```python
from build123d import *
from OCP.BRepFilletAPI import BRepFilletAPI_MakeChamfer

# Parameters (mm, degrees)
BOSS_EXTRUDE1_DEPTH = 9.8
CUT_EXTRUDE1_START  = -4.1
CUT_EXTRUDE1_DEPTH  = 4.1
SKETCH3_W           = 60.6
SKETCH3_H           = 100.9
CUT_EXTRUDE2_DEPTH  = 6.3
SKETCH4_W           = 1.6
SKETCH4_H           = 58.7
SKETCH4_W_2         = 45.4
SKETCH4_H_2         = 71.1
CUT_EXTRUDE3_DEPTH  = 71.319005255
BOSS_EXTRUDE3_START = -4.5
BOSS_EXTRUDE3_DEPTH = 4.5
CUT_EXTRUDE4_START  = -2.5
CUT_EXTRUDE4_DEPTH  = 4
CUT_EXTRUDE5_START  = -1.7
CUT_EXTRUDE5_DEPTH  = 3.1
FILLET1_R           = 6
FILLET2_R           = 4
FILLET3_R           = 2.5
CUT_EXTRUDE6_DEPTH  = 1.5
CHAMFER1_SIZE       = 1
CHAMFER2_SIZE       = 0.6
CHAMFER2_SIZE2      = 0.651920241
CHAMFER2_SIZE2_2    = 0.691050664
FILLET4_R           = 2


# Read off the part's stored shape, not the designer's step: Boss-Extrude3
with BuildPart() as part:
    # Sketch1 → Boss-Extrude1 (new body)
    with BuildSketch(Plane.XY):
        with BuildLine():
            ThreePointArc((-38, 0), (-37.524874157, -29.190462912), (-36.1, -58.35))
            Line((-36.1, -58.35), (36.1, -58.35))
            ThreePointArc((36.1, -58.35), (37.524874157, -29.190462912), (38, 0))
            ThreePointArc((38, 0), (37.524874157, 29.190462912), (36.1, 58.35))
            Line((36.1, 58.35), (-36.1, 58.35))
            ThreePointArc((-36.1, 58.35), (-37.524874157, 29.190462912), (-38, 0))
        make_face()
    extrude(amount=BOSS_EXTRUDE1_DEPTH)

    # Sketch2 → Cut-Extrude1 (cut)
    with BuildSketch(Plane.XY.offset(9.8).offset(CUT_EXTRUDE1_START)):
        with BuildLine():
            ThreePointArc((36.1, -58.35), (38, 0), (36.1, 58.35))
            Line((36.1, 58.35), (-36.1, 58.35))
            ThreePointArc((-36.1, 58.35), (-38, 0), (-36.1, -58.35))
            Line((-36.1, -58.35), (36.1, -58.35))
        make_face()
        with BuildLine():
            Line((-32, 54.5), (32, 54.5))
            ThreePointArc((32, 54.5), (33.8, 0), (32, -54.5))
            Line((32, -54.5), (-32, -54.5))
            ThreePointArc((-32, -54.5), (-33.8, 0), (-32, 54.5))
        make_face(mode=Mode.SUBTRACT)
    extrude(amount=CUT_EXTRUDE1_DEPTH, mode=Mode.SUBTRACT)

    # Sketch3 → Cut-Extrude2 (cut)
    with BuildSketch(Plane.XY.offset(9.8)):
        with Locations((0, 0.65)):
            Rectangle(SKETCH3_W, SKETCH3_H)
    extrude(amount=-CUT_EXTRUDE2_DEPTH, mode=Mode.SUBTRACT)

    # Sketch4 → Cut-Extrude3 (cut, through all)
    with BuildSketch(Plane(origin=(0, 0, 0), x_dir=(-1, 0, 0), z_dir=(0, 0, -1))):
        with Locations((23.5, -3)):
            Rectangle(SKETCH4_W, SKETCH4_H)
        with Locations((0, 0.1)):
            Rectangle(SKETCH4_W_2, SKETCH4_H_2)
        with BuildLine():
            Line((-2.1, -43.35), (2.1, -43.35))
            ThreePointArc((2.1, -43.35), (3.8, -41.65), (2.1, -39.95))
            Line((2.1, -39.95), (-2.1, -39.95))
            ThreePointArc((-2.1, -39.95), (-3.8, -41.65), (-2.1, -43.35))
        make_face()
        with BuildLine():
            Line((1.7, 39.85), (1.7, 44.05))
            ThreePointArc((1.7, 44.05), (0, 45.75), (-1.7, 44.05))
            Line((-1.7, 44.05), (-1.7, 39.85))
            ThreePointArc((-1.7, 39.85), (0, 38.15), (1.7, 39.85))
        make_face()
    extrude(amount=-CUT_EXTRUDE3_DEPTH, mode=Mode.SUBTRACT)

    # Boss-Extrude3 outline → Boss-Extrude3 (add)
    with BuildSketch(Plane(origin=(0, 54.5, 0), x_dir=(1, 0, 0), z_dir=(0, 1, 0)).offset(BOSS_EXTRUDE3_START)):
        Polygon((0, -3.5), (0, -9.8), (5.5, -9.8), (6, -15), (22, -15), (22.5, -9.8), (26, -9.8), (26, -3.5), align=None)
    boss_extrude3 = extrude(amount=BOSS_EXTRUDE3_DEPTH)

    # Sketch7 → Cut-Extrude4 (cut)
    with BuildSketch(Plane(origin=(0, 54.5, 0), x_dir=(1, 0, 0), z_dir=(0, 1, 0)).offset(CUT_EXTRUDE4_START)):
        Polygon((19.5, -14), (8.5, -14), (7.346153846, 1), (20.653846154, 1), align=None)
    cut_extrude4 = extrude(amount=CUT_EXTRUDE4_DEPTH, mode=Mode.SUBTRACT)

    # Mirror3: Boss-Extrude3, Cut-Extrude4 across plane
    add(boss_extrude3.mirror(Plane(origin=(0, 0, 0), x_dir=(0, 0, 1), z_dir=(1, 0, 0))))
    add(cut_extrude4.mirror(Plane(origin=(0, 0, 0), x_dir=(0, 0, 1), z_dir=(1, 0, 0))), mode=Mode.SUBTRACT)

    # Sketch8 → Cut-Extrude5 (cut)
    with BuildSketch(Plane.XZ.offset(54.5).offset(CUT_EXTRUDE5_START)):
        Polygon((-20.75, -1), (-19.6, 8.2), (-8.4, 8.2), (-7.25, -1), align=None)
    cut_extrude5 = extrude(amount=CUT_EXTRUDE5_DEPTH, mode=Mode.SUBTRACT)

    # Mirror4: Cut-Extrude5 across plane
    add(cut_extrude5.mirror(Plane(origin=(0, 0, 0), x_dir=(0, 0, 1), z_dir=(1, 0, 0))), mode=Mode.SUBTRACT)

    # Fillet1
    fillet1_edges = [part.edges().sort_by_distance(p)[0] for p in [
        (36.1, 58.35, 2.85),
        (36.1, -58.35, 2.85),
        (-36.1, -58.35, 2.85),
        (-36.1, 58.35, 2.85),
    ]]
    fillet(fillet1_edges, radius=FILLET1_R)

    # Fillet2
    fillet2_edges = [part.edges().sort_by_distance(p)[0] for p in [
        (-30.3, -49.8, 6.65),
        (-30.3, 51.1, 6.65),
        (30.3, 51.1, 6.65),
        (30.3, -49.8, 6.65),
    ]]
    fillet(fillet2_edges, radius=FILLET2_R)

    # Fillet3
    fillet3_edges = [part.edges().sort_by_distance(p)[0] for p in [
        (32, 54.5, 7.75),
        (-32, 54.5, 7.75),
        (-32, -54.5, 7.75),
        (32, -54.5, 7.75),
    ]]
    fillet(fillet3_edges, radius=FILLET3_R)

    # Sketch10 → Cut-Extrude6 (cut)
    with BuildSketch(Plane.XY.offset(5.7)):
        with BuildLine():
            Line((30.460657239, 55.35), (-30.460657239, 55.35))
            ThreePointArc((-30.460657239, 55.35), (-32.518710973, 54.532753955), (-33.455473858, 52.526276553))
            ThreePointArc((-33.455473858, 52.526276553), (-35, 0), (-33.455473858, -52.526276553))
            ThreePointArc((-33.455473858, -52.526276553), (-33.188926222, -53.597617073), (-32.552904835, -54.5))
            Line((-32.552904835, -54.5), (-34.974801677, -54.5))
            ThreePointArc((-34.974801677, -54.5), (-35.303180702, -53.59497651), (-35.45201827, -52.643794255))
            ThreePointArc((-35.45201827, -52.643794255), (-37, 0), (-35.45201827, 52.643794255))
            ThreePointArc((-35.45201827, 52.643794255), (-33.890746795, 55.987923259), (-30.460657239, 57.35))
            Line((-30.460657239, 57.35), (30.460657239, 57.35))
            ThreePointArc((30.460657239, 57.35), (33.890746795, 55.987923259), (35.45201827, 52.643794255))
            ThreePointArc((35.45201827, 52.643794255), (37, 0), (35.45201827, -52.643794255))
            ThreePointArc((35.45201827, -52.643794255), (35.303180702, -53.59497651), (34.974801677, -54.5))
            Line((34.974801677, -54.5), (32.552904835, -54.5))
            ThreePointArc((32.552904835, -54.5), (33.188926222, -53.597617073), (33.455473858, -52.526276553))
            ThreePointArc((33.455473858, -52.526276553), (35, 0), (33.455473858, 52.526276553))
            ThreePointArc((33.455473858, 52.526276553), (32.518710973, 54.532753955), (30.460657239, 55.35))
        make_face()
    extrude(amount=-CUT_EXTRUDE6_DEPTH, mode=Mode.SUBTRACT)

    # Chamfer1
    # the kernel refuses this chamfer: 1 mm, written as the material it takes off along each edge
    with BuildSketch(Plane(origin=(32.228209132, -54.5, 9.8), x_dir=(0, 0.9996219169112968, 0.02749587661058555), z_dir=(-1, 0, 0))) as chamfer1_piece_1:
        Polygon((CHAMFER1_SIZE * 0.999621916911, CHAMFER1_SIZE * 0.0274958766106), (-CHAMFER1_SIZE * 0.0274958766106, CHAMFER1_SIZE * 0.999621916911), (0, 0), align=None)
    extrude(amount=64.456418264, mode=Mode.SUBTRACT)

    # Chamfer2: one chamfer whose edges measure the first distance from different faces: ONE call of the kernel's chamfer builder (chamfer() names one face for all edges)
    chamfer2_edges_1 = [part.edges().sort_by_distance(p)[0] for p in [
        (14, 52, 0),
        (14, 56, 0),
        (-14, 52, 0),
        (-14, 56, 0),
        (-14, -52.8, 0),
        (-14, -55.9, 0),
        (14, -52.8, 0),
        (14, -55.9, 0),
        (0, -58.35, 0),
        (0, 58.35, 0),
        (38, 0, 0),
        (-38, 0, 0),
        (34.576764706, 56.715507911, 0),
        (-34.576764706, 56.715507911, 0),
        (34.576764706, -56.715507911, 0),
        (-34.576764706, -56.715507911, 0),
        (1.7, 41.95, 0),
        (-1.7, 41.95, 0),
        (0, 45.75, 0),
        (0, 38.15, 0),
        (0, -39.95, 0),
        (0, -43.35, 0),
        (-3.8, -41.65, 0),
        (3.8, -41.65, 0),
        (-23.5, -32.35, 0),
        (-22.7, -33.9, 0),
        (0, 35.65, 0),
        (-22.7, 31, 0),
        (-23.5, 26.35, 0),
        (-24.3, -3, 0),
        (22.7, 0.1, 0),
        (0, -35.45, 0),
    ]]
    chamfer2_edges_2 = [part.edges().sort_by_distance(p)[0] for p in [
        (20.576923077, 54, 0),
        (7.423076923, 54, 0),
    ]]
    chamfer2_side_2 = [part.faces().sort_by_distance(p)[0] for p in [
        (0, -56.957344623, 0),
    ]]
    chamfer2_edges_3 = [part.edges().sort_by_distance(p)[0] for p in [
        (-20.576923077, 54, 0),
    ]]
    chamfer2_side_3 = [part.faces().sort_by_distance(p)[0] for p in [
        (-20.098958851, 53.596109806, 6.213534938),
    ]]
    chamfer2_edges_4 = [part.edges().sort_by_distance(p)[0] for p in [
        (-7.423076923, 54, 0),
    ]]
    chamfer2_side_4 = [part.faces().sort_by_distance(p)[0] for p in [
        (-7.901041149, 53.596109806, 6.213534938),
    ]]
    chamfer2_edges_5 = [part.edges().sort_by_distance(p)[0] for p in [
        (-7.375, -54.35, 0),
        (-20.625, -54.35, 0),
    ]]
    chamfer2_side_5 = [part.faces().sort_by_distance(p)[0] for p in [
        (0, -56.957344623, 0),
    ]]
    chamfer2_edges_6 = [part.edges().sort_by_distance(p)[0] for p in [
        (20.625, -54.35, 0),
    ]]
    chamfer2_side_6 = [part.faces().sort_by_distance(p)[0] for p in [
        (20.169382984, -54.214279197, 3.644936131),
    ]]
    chamfer2_edges_7 = [part.edges().sort_by_distance(p)[0] for p in [
        (7.375, -54.35, 0),
    ]]
    chamfer2_side_7 = [part.faces().sort_by_distance(p)[0] for p in [
        (7.830617016, -54.214279197, 3.644936131),
    ]]
    chamfer2 = BRepFilletAPI_MakeChamfer(part.part.solid().wrapped)
    for e in chamfer2_edges_1:
        chamfer2.Add(CHAMFER2_SIZE, e.wrapped)
    for e in chamfer2_edges_2:
        chamfer2.Add(CHAMFER2_SIZE, CHAMFER2_SIZE2, e.wrapped, chamfer2_side_2[0].wrapped)  # the first distance lies on this face
    for e in chamfer2_edges_3:
        chamfer2.Add(CHAMFER2_SIZE, CHAMFER2_SIZE2, e.wrapped, chamfer2_side_3[0].wrapped)  # the first distance lies on this face
    for e in chamfer2_edges_4:
        chamfer2.Add(CHAMFER2_SIZE, CHAMFER2_SIZE2, e.wrapped, chamfer2_side_4[0].wrapped)  # the first distance lies on this face
    for e in chamfer2_edges_5:
        chamfer2.Add(CHAMFER2_SIZE, CHAMFER2_SIZE2_2, e.wrapped, chamfer2_side_5[0].wrapped)  # the first distance lies on this face
    for e in chamfer2_edges_6:
        chamfer2.Add(CHAMFER2_SIZE, CHAMFER2_SIZE2_2, e.wrapped, chamfer2_side_6[0].wrapped)  # the first distance lies on this face
    for e in chamfer2_edges_7:
        chamfer2.Add(CHAMFER2_SIZE, CHAMFER2_SIZE2_2, e.wrapped, chamfer2_side_7[0].wrapped)  # the first distance lies on this face
    add(Compound.cast(chamfer2.Shape()), mode=Mode.REPLACE)

    # Fillet4
    fillet4_edges = [part.edges().sort_by_distance(p)[0] for p in [
        (5.5, 52.25, 9.8),
        (22.5, 52.25, 9.8),
        (22, 52.25, 15),
        (6, 52.25, 15),
        (-22.5, 52.25, 9.8),
        (-5.5, 52.25, 9.8),
        (-6, 52.25, 15),
        (-22, 52.25, 15),
    ]]
    fillet(fillet4_edges, radius=FILLET4_R)


solid = part.part
```
CAD build for the part. Positions are in the model's coordinates, mm. A direction names the side the tool comes from. Give positions to 0.01 mm unless a question says otherwise; leave off trailing zeros. Use one line per item in the form item = value.
Item 1: Flat gauge pins, fed straight in: pin 1 (7 mm diameter, centred on y = 2, z = 5.5, fed in from -X); pin 2 (0.9 mm diameter, centred on x = 12, y = -54, fed in from -Z); pin 3 (2 mm diameter, centred on y = -10, z = 2.5, fed in from +X); pin 4 (1.9 mm diameter, centred on x = 4.5, z = 7, fed in from +Y). Where does each tip first touch, or does it go through?
Determined:
pin_1 = -38
pin_2 = 8.2
pin_3 = 37.95
pin_4 = 54.5
Item 2: Drill centre lines: probe 1 along Y at (x, z) = (-11.5, 3); probe 2 along Y at (x, z) = (-5.5, 7.25); probe 3 along X at (y, z) = (1.5, 8.5). Where is each one in solid material? Low to high. Write a range as from..to.
Determined:
probe_1 = -58.35..-55.9, -52.8..-35.45, 35.65..52, 56..58.35
probe_2 = -54.5..-49.8, 50..54.5
probe_3 = -33.8..-30.3, 30.3..33.8
Item 3: Slice it at A-A (x = 0). Count the separate pieces of the cut face and the enclosed holes in it, plus the area to 3 significant figures.
Determined:
separate_pieces = 4
enclosed_holes = 0
area = 191 mm2
Item 4: Which spindle directions (+Z, -Z, +X, -X, +Y, -Y) get a long thin tool onto all of the face, cutting with end or side? Do faces 1 (the face through (0, -43.35, 2)), 2 (the face through (31.35, 53.84, 7.78)), 3 (the face through (-30.3, 0, 7)), 4 (the face through (34.623, 56.672, 3.186)), 5 (the face through (-7.833, -54.328, 3.661)). Say none if no direction does.
Determined:
face_1 = +Z, -Z
face_2 = +Z, +X, +Y
face_3 = +Z
face_4 = +Z, -Z, +X, +Y
face_5 = -Z
Item 5: Two-plate mould, pull along X, no slides. Class faces 6 (the face through (31.39, -53.8, 7.78)), 7 (the face through (-34.53, 56.76, 3.19)), 8 (the face through (-0.04, 45.91, 0.44)): pulls with the +X half, pulls with the -X half, needs draft (parallel to the pull), parting line crosses it, or undercut.
Determined:
face_6 = pulls with the +X half
face_7 = pulls with the -X half
face_8 = undercut
